For this review, take the finished solid that the model builds, in its own axes (mm). A direction names the side the tool comes from. Round coordinates to 2 decimals unless told otherwise and drop trailing zeros. Loops run counter-clockwise (first coordinate to the right, second up) from the corner with the lowest first, then second, coordinate; pieces in that order, holes last.
1. Clearance check with flat-ended pins moving along their axes: pin 1 Ø1 at (x, y) = (15.5, 29) entering from +Z; pin 2 Ø5 at (x, z) = (-1, 5.5) entering from +Y. State where each tip first meets the part, or that it passes through.
2. Tool access review of faces 1 (the flat face through (0, 0, 5)), 2 (the flat face through (-16.807, 22.165, 4.93)): name each direction out of +Z, -Z, +X, -X, +Y, -Y from which nothing blocks a thin tool from reaching the whole face with its end or side.
3. Consider section C-C on y = 5.5. State the section outline as (x, z) points, then the cut area to 3 significant figures.
4. To check wall thickness, follow line 1 along Y through (x, z) = (-5.5, 5.75); line 2 along X through (y, z) = (15, 6.5); line 3 along X through (y, z) = (31, 1.5). State the ranges of each line that lie inside material, in increasing order.
5. Consider section D-D on x = 6. State the section outline as (y, z) points, then the cut area to 3 significant figures.
6. Consider section A-A on z = 5.5. State the section outline as (x, y) points.
7. Draft analysis for pull direction X (two halves, no side actions). For faces 3 (the flat face through (0, 2, 0)), 4 (the cylindrical face through (-13.35, 6.26, 5.07)), 5 (the flat face through (25, 18, 5)), 6 (the flat face through (-25, 19, 5)), state which applies: released by +X, released by -X, zero draft, split by the parting line, or undercut.
8. Consider section B-B on y = 23. State the section outline as (x, z) points, then the cut area to 3 significant figures.
from build123d import *

# Parameters (mm, degrees)
EXTRUDE_1_DEPTH = 10
FILLET_1_R      = 3.5
FILLET_2_R      = 7


with BuildPart() as part:
    # 草图1 → 凸台-拉伸1 (new body)
    with BuildSketch(Plane(origin=(0, 0, 0), x_dir=(-1, 0, 0), z_dir=(0, 0, -1))):
        Polygon((25, 0), (-25, 0), (-25, 37), (-18.290755601, 37), (-15.040755601, 4.5), (15.040755601, 4.5), (18.290755601, 37), (25, 37), align=None)
    extrude(amount=-EXTRUDE_1_DEPTH)

    # 圆角1
    fillet_1_edges = [part.edges().sort_by_distance(p)[0] for p in [
        (-18.290755601, 37, 5),
        (18.290755601, 37, 5),
    ]]
    fillet(fillet_1_edges, radius=FILLET_1_R)

    # 圆角2
    fillet_2_edges = [part.edges().sort_by_distance(p)[0] for p in [
        (-15.040755601, 4.5, 5),
        (15.040755601, 4.5, 5),
    ]]
    fillet(fillet_2_edges, radius=FILLET_2_R)


solid = part.part
Resolved:
1. pin 1: passes through
1. pin 2: stops at y = 4.5
2. face 1: +Z, -Z, +X, -X, -Y
2. face 2: +Z, -Z, +Y
3. outline: (-25, 0) - (-12.31, 0) - (-12.31, 10) - (-25, 10) - close; (12.31, 0) - (25, 0) - (25, 10) - (12.31, 10) - close
3. area: 254 mm2
4. line 1: y = 0 to 4.5
4. line 2: x = -25 to -16.09, 16.09 to 25
4. line 3: x = -25 to -17.69, 17.69 to 25
5. outline: (0, 0) - (4.5, 0) - (4.5, 10) - (0, 10) - close
5. area: 45.0 mm2
6. outline: (-25, 0) - (25, 0) - (25, 37) - (21.46, 37) arc R3.5 ccw to (17.98, 33.85) - (15.67, 10.8) arc R7 cw to (8.71, 4.5) - (-8.71, 4.5) arc R7 cw to (-15.67, 10.8) - (-17.98, 33.85) arc R3.5 ccw to (-21.46, 37) - (-25, 37) - close
7. face 3: zero draft
7. face 4: undercut
7. face 5: released by +X
7. face 6: released by -X
8. outline: (-25, 0) - (-16.89, 0) - (-16.89, 10) - (-25, 10) - close; (16.89, 0) - (25, 0) - (25, 10) - (16.89, 10) - close
8. area: 162 mm2
